Autodesk Fusion 360 part; units mm, degrees
sketch "Sketch1" plane through (0, 0, 0) normal (0, 0, 1) x (1, 0, 0)
  line L0 (-28.5903, -0.0704) -> (11.5163, -0.0704)
  line L1 (11.5163, -0.0704) -> (11.5163, 24.0596)
  line L2 (11.5163, 24.0596) -> (-28.5903, 24.0596)
  line L3 (-28.5903, 24.0596) -> (-28.5903, -0.0704)
  line L4 (-8.537, 24.0596) -> (-8.537, -0.0704) construction
  line L5 (-28.5903, 3.0284) -> (11.5163, 3.0284) construction
  circle A0 centre (-25.4661, 21.0116) radius 1.5621
  circle A1 centre (8.8908, 21.0116) radius 1.5621
  circle A2 centre (8.8908, 3.0366) radius 1.5621
  circle A3 centre (-25.4661, 3.0366) radius 1.5621
  line L6 (-25.4661, 21.0116) -> (-25.4661, 3.0366) construction
  line L7 (-25.4661, 3.0366) -> (8.8908, 3.0366) construction
  line L8 (8.8908, 3.0366) -> (8.8908, 21.0116) construction
  line L9 (8.8908, 21.0116) -> (-25.4661, 21.0116) construction
  line L10 (-17.572, 16.5219) -> (-0.0282, 16.5219) construction
  line L11 (-13.6343, 7.2364) -> (-11.3582, 3.0366) construction
  line L12 (-5.7345, 3.0366) -> (-3.185, 7.5867) construction
  circle A4 centre (-8.537, 17.0283) radius 0.9998
  circle A5 centre (-4.0328, 4.0283) radius 0.9998
  circle A6 centre (-13.0328, 4.0283) radius 0.9998
  line L13 (-9.4819, 17.355) -> (-13.9777, 4.355) construction
  line L14 (-7.5923, 17.3556) -> (-3.0881, 4.3556) construction
  line L15 (-9.77, 16.5219) -> (-13.2356, 6.5009)
  line L16 (-7.3035, 16.5219) -> (-3.8169, 6.459)
  line L17 (-11.3582, 3.0366) -> (-5.7345, 3.0366)
  arc A7 (-11.3582, 3.0366) -> (-13.2356, 6.5009) centre (-14.3377, 3.6627) ccw
  arc A8 (-3.8169, 6.459) -> (-5.7345, 3.0366) centre (-2.8758, 3.6832) ccw
  arc A9 (-9.8839, 16.1927) -> (-7.1785, 16.1614) centre (-8.5198, 17.1617) ccw
  point P0 (-13.2356, 6.5009)
  point P1 (-3.8169, 6.459)
  dimension "d1" = 40.1066
  dimension "d2" = 24.13
  dimension "d12" = 3.0988
  dimension "d15" = 3.1242
  dimension "d16" = 3.048
  dimension "d17" = 3.1242
  dimension "d25" = 13
  dimension "d26" = 9
  dimension "d27" = 13
  dimension "d28" = 4.4958
  dimension "d29" = 4.5042
extrude "Extrude1" add sketch "Sketch1" along normal blind 1.5748
Check sheet for the modelled part. Datum: model origin and axes. Units: mm. A direction names the side the tool comes from. Round coordinates to 2 decimals unless told otherwise and drop trailing zeros. Loops run counter-clockwise (first coordinate to the right, second up) from the corner with the lowest first, then second, coordinate; pieces in that order, holes last. Notation, with made-up numbers: M -25,14 L 29,14 A29 ccw 29,34 Z; hole C -15.5,-3 d5. An arc over 180 degrees is marked long. One line per item, written item: value.
(1) Sectioned sample at C-C, the plane z = 0.65. Count the separate pieces of the cut face and the enclosed holes in it, then the cut area to 3 significant figures.
Computed values:
separate pieces: 1
enclosed holes: 8
area: 848 mm^2
(2) Sectioned sample at D-D, the plane x = -25. Record the cut outline in (y, z).
Computed values:
outline: M -0.07,0 L 1.55,0 L 1.55,1.57 L -0.07,1.57 Z; M 4.53,0 L 19.52,0 L 19.52,1.57 L 4.53,1.57 Z; M 22.5,0 L 24.06,0 L 24.06,1.57 L 22.5,1.57 Z
(3) Sectioned sample at B-B, the plane x = -12.5. Record the cut outline in (y, z).
Computed values:
outline: M -0.07,0 L 3.18,0 L 3.18,1.57 L -0.07,1.57 Z; M 4.87,0 L 6.09,0 L 6.09,1.57 L 4.87,1.57 Z; M 8.63,0 L 24.06,0 L 24.06,1.57 L 8.63,1.57 Z
(4) Depth check by flat-ended pin: pin 1 Ø1.8 at (x, y) = (-4.03, 4.03) entering from +Z. Enter the tip coordinate at first touch or a pass-through.
Computed values:
pin 1: passes through
(5) Sectioned sample at A-A, the plane y = 17.5. Record the cut outline in (x, z).
Computed values:
outline: M -28.59,0 L -9.42,0 L -9.42,1.57 L -28.59,1.57 Z; M -7.66,0 L 11.52,0 L 11.52,1.57 L -7.66,1.57 Z
(6) Release check for a two-part mould opening along Y. For faces 3 (the face through (-4.25, 5.004, 0.776)), 4 (the face through (-28.59, 12, 1)), 5 (the face through (-8, 24.06, 1)) record: +Y half, -Y half, draft (parallel to the pull), parting line (faces both ways), or undercut.
Computed values:
face 3: undercut
face 4: draft
face 5: +Y half
(7) Thickness scan on line 1 (X direction, y = 21, z = 0.6); line 2 (X direction, y = 1.75, z = 1.25); line 3 (X direction, y = 4, z = 1.05). Record the ranges inside material, lowest first.
Computed values:
line 1: x = -28.59 to -27.03, -23.9 to 7.33, 10.45 to 11.52
line 2: x = -28.59 to -26.35, -24.58 to 8, 9.78 to 11.52
line 3: x = -28.59 to -26.7, -24.24 to -14.03, -12.03 to -11.31, -5.79 to -5.03, -3.03 to 7.66, 10.12 to 11.52
(8) Access from +Z, -Z, +X, -X, +Y, -Y to the whole of each face (thin tool, end or side, straight path). Record for faces 1 (the face through (-11.536, 11.415, 0.776)), 2 (the face through (11.516, 12, 1)).
Computed values:
face 1: +Z, -Z
face 2: +Z, -Z, +X, +Y, -Y
